Check sheet for the drawn part. Datum: minimum x, y, z corner. Units: mm. A direction names the side the tool comes from. Coordinates: 2 decimals unless noted, no trailing zeros. Write each loop counter-clockwise with the first axis right and the second up, starting at its lowest first coordinate (ties: lowest second). Pieces come first, ordered by that corner, then holes. Notation, with made-up numbers: (-35, -30.5) -> (-24, -30.5) arc R21 cw to (-24, -6.5) -> close; hole circle Ø7 at (41, 37). An arc over 180 degrees is marked (long way). Answer in a Markdown table with one row per item.
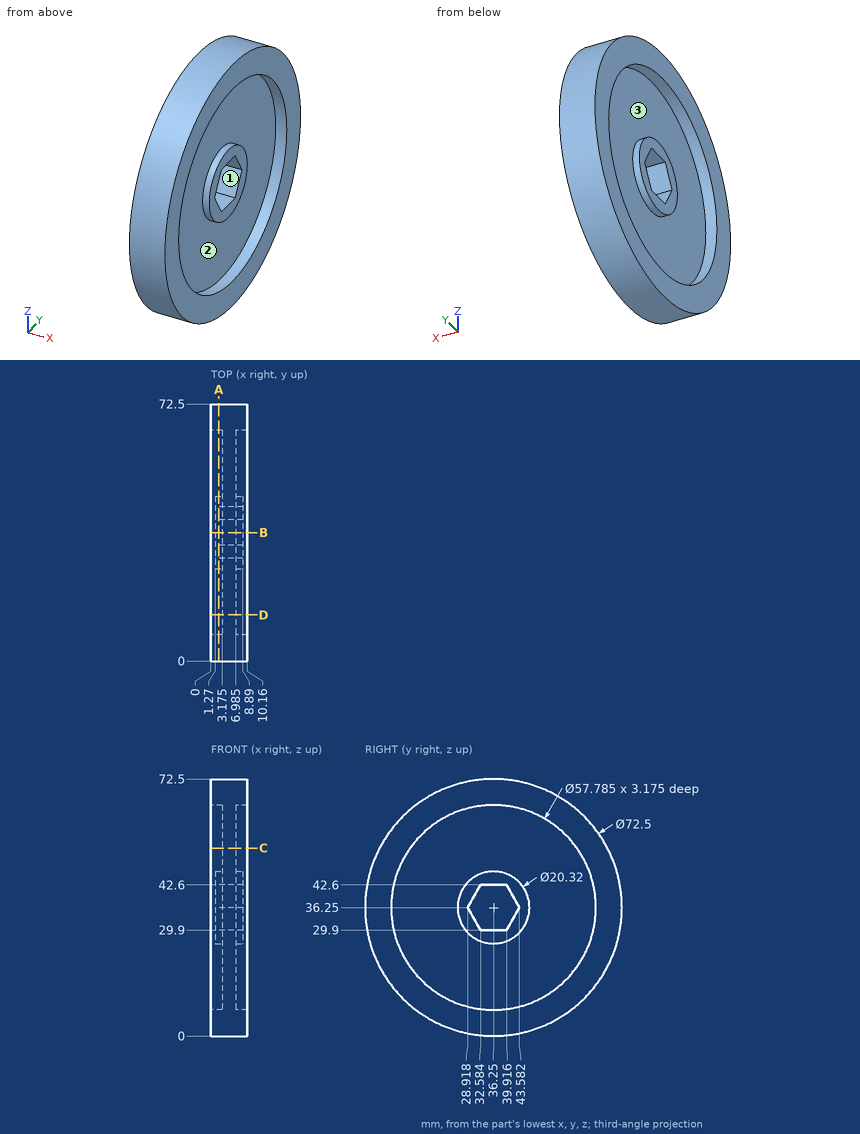
1. Go/stop test with flat-tipped pins: pin 1 (12 mm diameter, centred on y = 43.5, z = 22, fed in from +X); pin 2 (6 mm diameter, centred on x = 7, y = 37.5, fed in from +Z); pin 3 (2 mm diameter, centred on x = 3.5, y = 37, fed in from -Z). Record where each tip stops, or that it passes through.
Findings below:
| item | result |
|---|---|
| pin 1 | stops at x = 8.89 |
| pin 2 | stops at z = 72.5 |
| pin 3 | stops at z = 0 |
2. Sectioned sample at C-C, the plane z = 53. Record the cut outline in (x, y) (1 decimal).
Findings below:
| item | result |
|---|---|
| outline | (0, 4.1) -> (10.2, 4.1) -> (10.2, 12.7) -> (7, 12.7) -> (7, 59.8) -> (10.2, 59.8) -> (10.2, 68.4) -> (0, 68.4) -> (0, 59.8) -> (3.2, 59.8) -> (3.2, 12.7) -> (0, 12.7) -> close |
3. Access from +Z, -Z, +X, -X, +Y, -Y to the whole of each face (thin tool, end or side, straight path). Record for the marked faces 1, 2 and 3.
Findings below:
| item | result |
|---|---|
| face 1 | +X, -X |
| face 2 | +X |
| face 3 | -X |
4. Material ranges on probe 1 along Z at (x, y) = (2.3, 36.25); probe 2 along Z at (x, y) = (9.4, 36.25); probe 3 along Y at (x, z) = (8.5, 17) (1 decimal), recorded low to high. Write a range as from..to.
Findings below:
| item | result |
|---|---|
| probe 1 | z = 0..7.36, 26.09..29.9, 42.6..46.41, 65.14..72.5 |
| probe 2 | z = 0..7.36, 65.14..72.5 |
| probe 3 | y = 5.5..14.7, 57.8..67 |
5. Sectioned sample at A-A, the plane x = 2.25. Count the separate pieces of the cut face and the enclosed holes in it, and give its area (3 significant figures).
Findings below:
| item | result |
|---|---|
| separate pieces | 2 |
| enclosed holes | 2 |
| area | 1,690 mm² |
6. Sectioned sample at B-B, the plane y = 36.25. Record the cut outline in (x, z) (1 decimal).
Findings below:
| item | result |
|---|---|
| outline | (0, 0) -> (10.2, 0) -> (10.2, 7.4) -> (7, 7.4) -> (7, 26.1) -> (8.9, 26.1) -> (8.9, 29.9) -> (1.3, 29.9) -> (1.3, 26.1) -> (3.2, 26.1) -> (3.2, 7.4) -> (0, 7.4) -> close; (0, 65.1) -> (3.2, 65.1) -> (3.2, 46.4) -> (1.3, 46.4) -> (1.3, 42.6) -> (8.9, 42.6) -> (8.9, 46.4) -> (7, 46.4) -> (7, 65.1) -> (10.2, 65.1) -> (10.2, 72.5) -> (0, 72.5) -> close |
7. Sectioned sample at D-D, the plane y = 13. Record the cut outline in (x, z) (1 decimal).
Findings below:
| item | result |
|---|---|
| outline | (0, 8.4) -> (10.2, 8.4) -> (10.2, 19.1) -> (7, 19.1) -> (7, 53.4) -> (10.2, 53.4) -> (10.2, 64.1) -> (0, 64.1) -> (0, 53.4) -> (3.2, 53.4) -> (3.2, 19.1) -> (0, 19.1) -> close |
